from build123d import *

# Parameters (mm, degrees)
BOSS_EXTRUDE3_DEPTH           = 30
BOSS_EXTRUDE3_DEPTH_BACK      = 30
BOSS_EXTRUDE4_DEPTH           = 15
BOSS_EXTRUDE4_DEPTH_BACK      = 15
BOSS_EXTRUDE5_DEPTH           = 15
BOSS_EXTRUDE5_DEPTH_BACK      = 15
FILLET1_R                     = 10
CBORE_FOR_M3_SHCS1_AT_2_COUNT = 2
CBORE_FOR_M3_SHCS1_AT_2_PITCH = 125
LPATTERN1_COUNT               = 2
LPATTERN1_PITCH               = 20
LPATTERN1_COL_COUNT           = 2
LPATTERN1_COL_PITCH           = 20
FILLET2_R                     = 2
FILLET3_R                     = 3


with BuildPart() as part:
    # Sketch1 → Boss-Extrude3 (new, two sides: drawn at the far end of the back side and taken through both)
    with BuildSketch(Plane.XY.offset(-BOSS_EXTRUDE3_DEPTH_BACK)):
        with BuildLine():
            Line((-43.065388601, -36.056178761), (-70, -36.056178761))
            Line((-70, -36.056178761), (-70, -46.056178761))
            Line((-70, -46.056178761), (70, -46.056178761))
            Line((70, -46.056178761), (70, -36.056178761))
            Line((70, -36.056178761), (43.065388601, -36.056178761))
            Line((43.065388601, -36.056178761), (26.080681992, -36.056178761))
            Line((26.080681992, -36.056178761), (16.130777202, -36.056178761))
            ThreePointArc((16.130777202, -36.056178761), (0, -39.5), (-16.130777202, -36.056178761))
            Line((-16.130777202, -36.056178761), (-26.080681992, -36.056178761))
            Line((-26.080681992, -36.056178761), (-43.065388601, -36.056178761))
        make_face()
    extrude(amount=BOSS_EXTRUDE3_DEPTH + BOSS_EXTRUDE3_DEPTH_BACK)

    # Sketch1_6 → Boss-Extrude4 (add, two sides: drawn at the far end of the back side and taken through both)
    with BuildSketch(Plane.XY.offset(-BOSS_EXTRUDE4_DEPTH_BACK)):
        with BuildLine():
            ThreePointArc((-43.065388601, -11.208135645), (-36.737597653, -25.111728708), (-26.080681992, -36.056178761))
            Line((-26.080681992, -36.056178761), (-16.130777202, -36.056178761))
            ThreePointArc((-16.130777202, -36.056178761), (-33.146762281, -21.483532071), (-39.5, 0))
            Line((-39.5, 0), (-44.5, 0))
            ThreePointArc((-44.5, 0), (-44.139890081, -5.649787927), (-43.065388601, -11.208135645))
        make_face()
        with BuildLine():
            ThreePointArc((39.5, 0), (33.146762281, -21.483532071), (16.130777202, -36.056178761))
            Line((16.130777202, -36.056178761), (26.080681992, -36.056178761))
            ThreePointArc((26.080681992, -36.056178761), (36.737597653, -25.111728708), (43.065388601, -11.208135645))
            ThreePointArc((43.065388601, -11.208135645), (44.139890081, -5.649787927), (44.5, 0))
            Line((44.5, 0), (39.5, 0))
        make_face()
    extrude(amount=BOSS_EXTRUDE4_DEPTH + BOSS_EXTRUDE4_DEPTH_BACK)

    # Sketch1_7 → Boss-Extrude5 (add, two sides: drawn at the far end of the back side and taken through both)
    with BuildSketch(Plane.XY.offset(-BOSS_EXTRUDE5_DEPTH_BACK)):
        with BuildLine():
            Line((26.080681992, -36.056178761), (43.065388601, -36.056178761))
            Line((43.065388601, -36.056178761), (43.065388601, -11.208135645))
            ThreePointArc((43.065388601, -11.208135645), (36.737597653, -25.111728708), (26.080681992, -36.056178761))
        make_face()
        with BuildLine():
            Line((-43.065388601, -11.208135645), (-43.065388601, -36.056178761))
            Line((-43.065388601, -36.056178761), (-26.080681992, -36.056178761))
            ThreePointArc((-26.080681992, -36.056178761), (-36.737597653, -25.111728708), (-43.065388601, -11.208135645))
        make_face()
    extrude(amount=BOSS_EXTRUDE5_DEPTH + BOSS_EXTRUDE5_DEPTH_BACK)

    # Fillet1
    fillet1_edges = [part.edges().sort_by_distance(p)[0] for p in [
        (43.065388601, -36.056178761, 0),
        (-43.065388601, -36.056178761, 0),
    ]]
    fillet(fillet1_edges, radius=FILLET1_R)

    # Sketch4 → CBORE for M3 SHCS1 (revolve, cut)
    with BuildSketch(Plane(origin=(-62.5, -36.056178761, 0), x_dir=(0, 0, 1), z_dir=(1, 0, 0))):
        Polygon((0, 0), (0, 10), (1.7, 10), (1.7, 3), (3.25, 3), (3.25, 0.025), (3.275, 0), align=None)
    cbore_for_m3_shcs1 = revolve(axis=Axis((-62.5, -29.706178761, 0), (0, -1, 0)), mode=Mode.SUBTRACT)

    # CBORE for M3 SHCS1 at 2: CBORE for M3 SHCS1 ×2
    with Locations(*[(i * CBORE_FOR_M3_SHCS1_AT_2_PITCH, 0, 0) for i in range(1, CBORE_FOR_M3_SHCS1_AT_2_COUNT)]):
        add(cbore_for_m3_shcs1, mode=Mode.SUBTRACT)

    # LPattern1: CBORE for M3 SHCS1 ×2
    with Locations(*[(0, 0, -i * LPATTERN1_PITCH) for i in range(1, LPATTERN1_COUNT)]):
        add(cbore_for_m3_shcs1, mode=Mode.SUBTRACT)

    # LPattern1 copy 1 sketch → LPattern1 copy 1 (revolve, cut)
    with BuildSketch(Plane(origin=(62.5, -36.056178761, -20), x_dir=(0, 0, 1), z_dir=(1, 0, 0))):
        Polygon((0, 0), (0, 10), (1.7, 10), (1.7, 3), (3.25, 3), (3.25, 0.025), (3.275, 0), align=None)
    revolve(axis=Axis((62.5, -29.706178761, -20), (0, -1, 0)), mode=Mode.SUBTRACT)

    # LPattern1 col: CBORE for M3 SHCS1 ×2
    with Locations(*[(0, 0, i * LPATTERN1_COL_PITCH) for i in range(1, LPATTERN1_COL_COUNT)]):
        add(cbore_for_m3_shcs1, mode=Mode.SUBTRACT)

    # LPattern1 col copy 1 sketch → LPattern1 col copy 1 (revolve, cut)
    with BuildSketch(Plane(origin=(62.5, -36.056178761, 20), x_dir=(0, 0, 1), z_dir=(1, 0, 0))):
        Polygon((0, 0), (0, 10), (1.7, 10), (1.7, 3), (3.25, 3), (3.25, 0.025), (3.275, 0), align=None)
    revolve(axis=Axis((62.5, -29.706178761, 20), (0, -1, 0)), mode=Mode.SUBTRACT)

    # Fillet2
    fillet2_edges = [part.edges().sort_by_distance(p)[0] for p in [
        (-44.5, 0, 0),
        (-39.5, 0, 0),
        (44.5, 0, 0),
        (39.5, 0, 0),
    ]]
    fillet(fillet2_edges, radius=FILLET2_R)

    # Fillet3
    fillet3_edges = [part.edges().sort_by_distance(p)[0] for p in [
        (-70, -41.056178761, -30),
        (70, -41.056178761, 30),
        (-70, -41.056178761, 30),
        (70, -41.056178761, -30),
    ]]
    fillet(fillet3_edges, radius=FILLET3_R)


solid = part.part
Could you check a few things on this model? Use its own coordinates, in mm. A direction names the side the tool comes from. Give positions to 0.01 mm unless a question says otherwise; leave off trailing zeros. Write each loop counter-clockwise with the first axis right and the second up, starting at its lowest first coordinate (ties: lowest second). Pieces come first, ordered by that corner, then holes. Notation, with made-up numbers: (13, 37.5) - (59, 37.5) arc R27 cw to (59, 66.5) - close; hole circle Ø10 at (-3, -10.75). An arc over 180 degrees is marked (long way). Use CSV: the item, a comma, the result in double quotes. Start each with the question number.
Item 1: I want a section at B-B, the plane x = 62.5. Give the number of separate pieces and of enclosed holes in the cut face, then the cut area to 3 significant figures.
Item 2: If I drill on line 1 along Z through (x, y) = (62.5, -37.55); line 2 along Z through (x, y) = (-62.5, -41.75); line 3 along Y through (x, z) = (45, -17), over which ranges is the centre line in solid material (lowest first)?
Item 3: I want a section at C-C, the plane y = -8.5. Please give me the cut outline in (x, z).
Item 4: For faces 4 (the face through (59.278, -37.548, 19.577)), 5 (the face through (-37, -23, -15)), 6 (the face through (-37, -23, 15)), which set-ups out of +Z, -Z, +X, -X, +Y, -Y let a thin tool reach every point of the face, with its end or its side?
Item 5: If we mould it in two halves opening along Y, with no side actions, what happens to faces 1 (the face through (-61.1, -39.056, 18.6)), 2 (the face through (-44.004, -6.623, -0.21)), 3 (the face through (-64.697, -37.548, 17.605))? For each: pulls with the +Y half, pulls with the -Y half, needs draft (parallel to the pull), parting line crosses it, or undercut.
Item 6: I'm going to push flat-ended pins straight in: pin 1 (6 mm diameter, centred on x = -52.5, z = 8.5, fed in from +Y); pin 2 (2 mm diameter, centred on x = -62.5, z = -20, fed in from +Y); pin 3 (12 mm diameter, centred on y = -20.5, z = 2, fed in from -X); pin 4 (5 mm diameter, centred on x = -62.5, z = 0, fed in from +Y). Where does each tip first touch, or does it pass through?
Item 7: I want a section at D-D, the plane z = 25. Please give me the cut outline in (x, y).
Item 8: I want a section at A-A, the plane z = -20. Please give me the cut outline in (x, y) (3 decimals).
Findings:
1,separate pieces,"4"
1,enclosed holes,"0"
1,area,"470 mm2"
2,line 1,"z = -30 to -23.25, -16.75 to -3.25, 3.25 to 16.75, 23.25 to 30"
2,line 2,"z = -30 to -21.7, -18.3 to -1.7, 1.7 to 18.3, 21.7 to 30"
2,line 3,"y = -46.06 to -36.06"
3,outline,"(-43.68, -15) - (-38.57, -15) - (-38.57, 15) - (-43.68, 15) - close; (38.57, -15) - (43.68, -15) - (43.68, 15) - (38.57, 15) - close"
4,face 4,"+Y"
4,face 5,"-Z, +X, -X, +Y"
4,face 6,"+Z, +X, -X, +Y"
5,face 1,"pulls with the +Y half"
5,face 2,"undercut"
5,face 3,"needs draft"
6,pin 1,"stops at y = -35.4"
6,pin 2,"passes through"
6,pin 3,"stops at x = -43.08"
6,pin 4,"stops at y = -39.06"
7,outline,"(-70, -46.06) - (70, -46.06) - (70, -36.06) - (16.13, -36.06) arc R39.5 cw to (-16.13, -36.06) - (-70, -36.06) - close"
8,outline,"(-70, -46.056) - (-64.2, -46.056) - (-64.2, -39.056) - (-65.75, -39.056) - (-65.75, -36.081) - (-65.775, -36.056) - (-70, -36.056) - close; (-60.8, -46.056) - (60.8, -46.056) - (60.8, -39.056) - (59.25, -39.056) - (59.25, -36.081) - (59.225, -36.056) - (16.131, -36.056) arc R39.5 cw to (-16.131, -36.056) - (-59.225, -36.056) - (-59.25, -36.081) - (-59.25, -39.056) - (-60.8, -39.056) - close; (64.2, -46.056) - (70, -46.056) - (70, -36.056) - (65.775, -36.056) - (65.75, -36.081) - (65.75, -39.056) - (64.2, -39.056) - close"
